Design review of the part built by this model. Coordinates are the model's own, in mm. A direction names the side the tool comes from. Give positions to 0.01 mm unless a question says otherwise; leave off trailing zeros.
```python
from build123d import *

# Parameters (mm, degrees)
FILLET1_R           = 1
SHELL4_T            = -0.3
SKETCH3_W           = 17.5
SKETCH3_H           = 17.5
BOSS_EXTRUDE1_DEPTH = 2
FILLET2_R           = 1
BOSS_EXTRUDE4_DEPTH = 8.5
FILLET4_R           = 0.5
CUT_EXTRUDE1_DEPTH  = 0.5


# Read off the part's stored shape, not the designer's step: Boss-Extrude4
with BuildPart() as part:
    # Sketch1 → Loft1 section 0
    with BuildSketch(Plane(origin=(0, 0, 0), x_dir=(0, 0, -1), z_dir=(1, 0, 0))):
        with BuildLine():
            Line((-8.25, -8.25), (8.25, -8.25))
            Line((8.25, -8.25), (8.25, 8.25))
            Line((8.25, 8.25), (-8.25, 8.25))
            Line((-8.25, 8.25), (-8.25, -8.25))
        make_face()
    # Sketch2 → Loft1 section 1
    with BuildSketch(Plane.ZY.offset(-8.5)):
        with BuildLine():
            Line((-7.25, -7.25), (7.25, -7.25))
            Line((7.25, -7.25), (7.25, 7.25))
            Line((7.25, 7.25), (-7.25, 7.25))
            Line((-7.25, 7.25), (-7.25, -7.25))
        make_face()
    loft()

    # Fillet1
    fillet1_edges = [part.edges().sort_by_distance(p)[0] for p in [
        (4.25, -7.75, -7.75),
        (4.25, -7.75, 7.75),
        (4.25, 7.75, -7.75),
        (4.25, 7.75, 7.75),
    ]]
    fillet(fillet1_edges, radius=FILLET1_R)

    # Shell4
    shell4_openings = [part.faces().sort_by_distance(p)[0] for p in [
        (8.5, 0, 0),
        (0, 0, 0),
    ]]
    offset(amount=SHELL4_T, openings=shell4_openings)

    # Sketch3 → Boss-Extrude1 (add)
    with BuildSketch(Plane(origin=(0, 0, 0), x_dir=(0, 0, -1), z_dir=(1, 0, 0))):
        Rectangle(SKETCH3_W, SKETCH3_H)
    extrude(amount=-BOSS_EXTRUDE1_DEPTH)

    # Fillet2
    fillet2_edges = [part.edges().sort_by_distance(p)[0] for p in [
        (-1, 8.75, -8.75),
        (-1, -8.75, -8.75),
        (-1, -8.75, 8.75),
        (-1, 8.75, 8.75),
    ]]
    fillet(fillet2_edges, radius=FILLET2_R)

    # Sketch5 → Revolve3 (revolve)
    with BuildSketch(Plane.XY, mode=Mode.PRIVATE) as revolve3_sk:
        with BuildLine():
            Line((0, 0), (0, 6))
            Line((0, 6), (5.5, 6))
            Line((5.5, 6), (5.5, 5))
            Line((5.5, 5), (8.5, 5))
            Line((8.5, 5), (8.5, 4.25))
            ThreePointArc((8.5, 4.25), (7.905950455, 3.193995394), (7.7, 2))
            Line((7.7, 2), (8.5, 1))
            Line((8.5, 1), (8.5, 0))
            Line((8.5, 0), (0, 0))
        make_face()
    revolve(revolve3_sk.sketch.rotate(Axis((8.5, 0, 0), (-1, 0, 0)), 90), axis=Axis((8.5, 0, 0), (-1, 0, 0)))

    # Boss-Extrude4 outline → Boss-Extrude4 (add)
    with BuildSketch(Plane(origin=(0, 0, 0), x_dir=(0, 0, -1), z_dir=(1, 0, 0))):
        with BuildLine():
            Line((7.25, -0.4), (7.25, 0.4))
            Line((7.25, 0.4), (4.983974318, 0.4))
            ThreePointArc((4.983974318, 0.4), (5, 0), (4.983974318, -0.4))
            Line((4.983974318, -0.4), (7.25, -0.4))
        make_face()
        with BuildLine():
            Line((-0.211850638, -4.995509915), (-0.188879124, -7.25))
            Line((-0.188879124, -7.25), (0.4, -7.25))
            Line((0.4, -7.25), (0.4, -4.983974318))
            ThreePointArc((0.4, -4.983974318), (0.094251329, -4.99911159), (-0.211850638, -4.995509915))
        make_face()
        with BuildLine():
            Line((-0.336622937, 7.25), (-0.313596871, 4.99015601))
            ThreePointArc((-0.313596871, 4.99015601), (0.04331199, 4.999812404), (0.4, 4.983974318))
            Line((0.4, 4.983974318), (0.4, 7.25))
            Line((0.4, 7.25), (-0.336622937, 7.25))
        make_face()
        with BuildLine():
            Line((-4.983974318, 0.4), (-7.25, 0.4))
            Line((-7.25, 0.4), (-7.25, -0.4))
            Line((-7.25, -0.4), (-4.983974318, -0.4))
            ThreePointArc((-4.983974318, -0.4), (-5, 0), (-4.983974318, 0.4))
        make_face()
    extrude(amount=BOSS_EXTRUDE4_DEPTH)

    # Sketch7 → Cut-Revolve2 (revolve, cut)
    with BuildSketch(Plane.XY):
        Polygon((-2, 0), (-2, 4.5), (-0.2, 4.5), (0, 4.85), (0.5, 4.85), (1.6375, 4.2), (6.7, 4.2), (6.7, 3.5), (3.1, 3.5), (3.1, 2.5), (6.7, 2.5), (6.7, 0), align=None)
    revolve(axis=Axis((6.7, 0, 0), (-1, 0, 0)), mode=Mode.SUBTRACT)

    # Fillet4
    fillet4_edges = [part.edges().sort_by_distance(p)[0] for p in [
        (3.1, -2.5, 0),
    ]]
    fillet(fillet4_edges, radius=FILLET4_R)

    # Sketch9 → Cut-Extrude1 (cut)
    with BuildSketch(Plane.ZY.offset(-6.7)):
        with BuildLine():
            Line((0.75, 2), (-0.75, 2))
            Line((-0.75, 2), (-0.75, -1.25))
            ThreePointArc((-0.75, -1.25), (-0.530330086, -1.780330086), (0, -2))
            ThreePointArc((0, -2), (0.303045763, -1.874474335), (0.428571429, -1.571428571))
            ThreePointArc((0.428571429, -1.571428571), (0.251190476, -1.039285714), (-0.21, -0.72))
            ThreePointArc((-0.21, -0.72), (0.45, -0.6), (0.75, 0))
            Line((0.75, 0), (0.75, 2))
        make_face()
    extrude(amount=-CUT_EXTRUDE1_DEPTH, mode=Mode.SUBTRACT)

    # Sketch10 → Cut-Revolve3 (revolve, cut)
    with BuildSketch(Plane.XY, mode=Mode.PRIVATE) as cut_revolve3_sk:
        Polygon((8.5, 0), (6.372171637, 0), (6.372171637, 0.75), (7.2, 0.75), (7.546410162, 0.15), (8.5, 0.15), align=None)
    revolve(cut_revolve3_sk.sketch.rotate(Axis((8.5, 0, 0), (-1, 0, 0)), 90), axis=Axis((8.5, 0, 0), (-1, 0, 0)), mode=Mode.SUBTRACT)


solid = part.part
```
(1) Clearance check with flat-ended pins moving along their axes: P1, Ø0.7, axis at x = 5, z = -6, coming from the -Y side; P2, Ø3, axis at x = 3.5, y = 3, coming from the +Z side; P3, Ø2.5, axis at x = 5.5, y = -6.5, coming from the -Z side. State where each tip first meets the part, or that it passes through.
Resolved:
P1: stops at y = -7.7
P2: stops at z = 8.01
P3: stops at z = -7.75
(2) Tool access review of faces 1 (the face through (2.79, -4.35, 4.13)), 2 (the face through (-1, 0, 8.75)), 3 (the face through (4.31, -0.1, -7.44)), 4 (the face through (-1.09, -0.59, -4.46)): name each direction out of +Z, -Z, +X, -X, +Y, -Y from which nothing blocks a thin tool from reaching the whole face with its end or side.
Resolved:
face 1: +X
face 2: +Z, +X, -X, +Y, -Y
face 3: none
face 4: -X
(3) To check wall thickness, follow L1, parallel to Z at x = -1.55, y = 0; L2, parallel to Z at x = 2, y = 2.25; L3, parallel to Z at x = 6, y = -2. State the ranges of each line that lie inside material, in increasing order.
Resolved:
L1: z = -8.75 to -4.5, 4.5 to 8.75
L2: z = -8.01 to -7.71, -5.56 to -3.55, 3.55 to 5.56, 7.71 to 8.01
L3: z = -7.54 to -7.24, -4.58 to -3.69, -2.87 to -1.5, 1.5 to 2.87, 3.69 to 4.58, 7.24 to 7.54
(4) Mouldability with a two-part tool opening along X and no side actions: class faces 5 (the face through (4.31, 7.44, -0.1)), 6 (the face through (8.5, -0.24, -0.21)), 7 (the face through (-1, -8.75, 0)) as pulls with the +X half, pulls with the -X half, needs draft (parallel to the pull), parting line crosses it, or undercut.
Resolved:
face 5: undercut
face 6: pulls with the +X half
face 7: needs draft
(5) Consider section A-A, the plane x = 2.75. Give the number of separate pieces and of enclosed holes in the cut face, then the cut area to 3 significant figures.
Resolved:
separate pieces: 2
enclosed holes: 2
area: 79.7 mm2
